Could you check a few things on this model? Use its own coordinates, in mm. Round coordinates to 2 decimals unless told otherwise and drop trailing zeros. Loops run counter-clockwise (first coordinate to the right, second up) from the corner with the lowest first, then second, coordinate; pieces in that order, holes last. Notation, with made-up numbers: M 38.25,-40 L 51.25,-40 A10 ccw 51.25,-29 Z; hole C 67,56.25 d4. An arc over 180 degrees is marked long. Return JSON: item names as keys, results as strings. Group by question number.
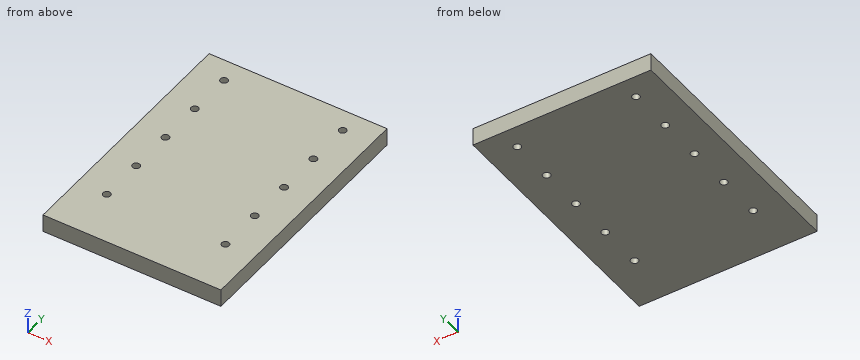
```python
from build123d import *

# Parameters (mm, degrees)
F1_DEPTH = 170
F3_D     = 5
F5_D     = 5


with BuildPart() as f1:
    # F0 (on Front) → F1 (new body)
    with BuildSketch(Plane.XZ):
        Polygon((0, 12), (0, 0), (120, 0), (120, 12), (66.9767542527, 12), align=None)
    extrude(amount=F1_DEPTH)

    # F3 (through all)
    with Locations(Plane.XY.offset(12)):
        with Locations((20, -15), (20, -45), (20, -75), (20, -105), (20, -135)):
            Hole(F3_D / 2)

    # F5 (through all)
    with Locations(Plane.XY.offset(12)):
        with Locations((100, -15), (100, -45), (100, -75), (100, -105), (100, -135)):
            Hole(F5_D / 2)


solid = f1.part
```
1. If we section it at A-A, the plane y = -75: Please give me the cut outline in (x, z).
2. I need wall thicknesses on probe 1 along Y at (x, z) = (100, 3.75); probe 2 along X at (y, z) = (-17, 10.5); probe 3 along Y at (x, z) = (21.5, 6.5). Which ranges of each line are inside material? Lowest first, please.
3. I'm going to push a flat-ended pin straight in: pin 1 Ø4 at (x, y) = (20, -105) entering from -Z. Where does the tip first touch, or does it pass through?
4. If we section it at B-B, the plane x = 100: Please give me the cut outline in (y, z).
Geometry results:
{
 "1": {"outline": "M 0,0 L 17.5,0 L 17.5,12 L 0,12 Z; M 22.5,0 L 97.5,0 L 97.5,12 L 22.5,12 Z; M 102.5,0 L 120,0 L 120,12 L 102.5,12 Z"},
 "2": {"probe 1": "-170 to -137.5, -132.5 to -107.5, -102.5 to -77.5, -72.5 to -47.5, -42.5 to -17.5, -12.5 to 0", "probe 2": "0 to 18.5, 21.5 to 98.5, 101.5 to 120", "probe 3": "-170 to -137, -133 to -107, -103 to -77, -73 to -47, -43 to -17, -13 to 0"},
 "3": {"pin 1": "through"},
 "4": {"outline": "M -170,0 L -137.5,0 L -137.5,12 L -170,12 Z; M -132.5,0 L -107.5,0 L -107.5,12 L -132.5,12 Z; M -102.5,0 L -77.5,0 L -77.5,12 L -102.5,12 Z; M -72.5,0 L -47.5,0 L -47.5,12 L -72.5,12 Z; M -42.5,0 L -17.5,0 L -17.5,12 L -42.5,12 Z; M -12.5,0 L 0,0 L 0,12 L -12.5,12 Z"}
}
